```python
from build123d import *

# Parameters (mm, degrees)
CYLINDER005_R     = 100
CYLINDER005_DEPTH = 350
FILLET010_1_R     = 100
FILLET010_2_R     = 30


with BuildPart() as part:
    # Cylinder005 → Cylinder005 (new body)
    with BuildSketch(Plane(origin=(-350, 0, 1730), x_dir=(1, 0, 0), z_dir=(0, 0, 1))):
        Circle(CYLINDER005_R)
    extrude(amount=CYLINDER005_DEPTH)

    # Fillet010 1
    fillet010_1_edges = [part.edges().sort_by_distance(p)[0] for p in [
        (-450, 0, 1730),
    ]]
    fillet(fillet010_1_edges, radius=FILLET010_1_R)

    # Fillet010 2
    fillet010_2_edges = [part.edges().sort_by_distance(p)[0] for p in [
        (-450, 0, 2080),
    ]]
    fillet(fillet010_2_edges, radius=FILLET010_2_R)


solid = part.part
```
Geometry check sheet. Reference: the model listing, model coordinates, mm. Give positions to 0.01 mm unless a question says otherwise; leave off trailing zeros. Write each loop counter-clockwise with the first axis right and the second up, starting at its lowest first coordinate (ties: lowest second). Pieces come first, ordered by that corner, then holes. Notation, with made-up numbers: (-33, 36) -> (3, 36) arc R26 ccw to (3, 66) -> close; hole circle Ø5 at (23.25, 51). An arc over 180 degrees is marked (long way). One line per question, with ' | ' between items.
Item 1: Sectioned sample at A-A, the plane x = -350. Record the boundary of the cut face in (y, z), plus the area to 3 significant figures.
Determined:
outline: (-100, 1830) arc R100 ccw to (100, 1830) -> (100, 2050) arc R30 ccw to (70, 2080) -> (-70, 2080) arc R30 ccw to (-100, 2050) -> close | area: 65,300 mm^2
Item 2: Sectioned sample at B-B, the plane y = 0. Record the boundary of the cut face in (x, z).
Determined:
outline: (-450, 1830) arc R100 ccw to (-250, 1830) -> (-250, 2050) arc R30 ccw to (-280, 2080) -> (-420, 2080) arc R30 ccw to (-450, 2050) -> close
Item 3: Depth check by flat-ended pin: pin 1 (1.5 mm diameter, centred on x = -312.5, z = 1944.5, fed in from +Y); pin 2 (3 mm diameter, centred on y = 59, z = 1967, fed in from +X); pin 3 (12 mm diameter, centred on x = -311.5, y = -40.5, fed in from -Z). Enter the tip coordinate at first touch or a pass-through.
Determined:
pin 1: y = 93 | pin 2: x = -268.18 | pin 3: z = 1743.33
Item 4: Sectioned sample at C-C, the plane z = 1978.5. Record the boundary of the cut face in (x, y), plus the area to 3 significant figures.
Determined:
outline: circle Ø200 at (-350, 0) | area: 31,400 mm^2
Item 5: Scan lines: line 1 along Y through (x, z) = (-312, 1994.5); line 2 along X through (y, z) = (43, 1815); line 3 along X through (y, z) = (58.5, 1957). Record each from-to range of solid material in increasing order.
Determined:
line 1: -92.5 to 92.5 | line 2: -439.03 to -260.97 | line 3: -431.1 to -268.9
